```python
from build123d import *

# Parameters (mm, degrees)
F0_W     = 9
F0_H     = 9
F0_H_2   = 432
F1_DEPTH = 18


# Not quite as in the source:
# - a feature names something its author has since deleted; it is built from what else it names


with BuildPart() as f1:
    # F0 (on Front) → F1 (new body)
    with BuildSketch(Plane.XZ):
        with Locations((-1095.5, 71.3756743552)):
            Rectangle(F0_W, F0_H)
        with BuildLine():
            Line((-973.3476458471, -374.1243256448), (-1054.6076226562, -374.1243256448))
            ThreePointArc((-1054.6076226562, -374.1243256448), (-1051.7483407187, -375.721921149), (-1051.265639742, -378.9614896944))
            Line((-1051.265639742, -378.9614896944), (-1098.3606008427, -558.954299013))
            ThreePointArc((-1098.3606008427, -558.954299013), (-1097.4812264988, -563.2754093644), (-1093.523436793, -565.219938755))
            Line((-1093.523436793, -565.219938755), (-1078.8076104242, -565.219938755))
            ThreePointArc((-1078.8076104242, -565.219938755), (-1076.2129629213, -564.4940239596), (-1074.371712623, -562.5270604893))
            Line((-1074.371712623, -562.5270604893), (-977.7835436484, -376.8172039105))
            ThreePointArc((-977.7835436484, -376.8172039105), (-975.94229335, -374.8502404402), (-973.3476458471, -374.1243256448))
        make_face()
        with BuildLine():
            Line((0, -365.1243256448), (-1091, -365.1243256448))
            Line((-1091, -365.1243256448), (-1091, -374.1243256448))
            Line((-1091, -374.1243256448), (-1055, -374.1243256448))
            ThreePointArc((-1055, -374.1243256448), (-1054.8038113281, -374.1191399972), (-1054.6076226562, -374.1243256448))
            Line((-1054.6076226562, -374.1243256448), (-973.3476458471, -374.1243256448))
            Line((-973.3476458471, -374.1243256448), (0, -374.1243256448))
            Line((0, -374.1243256448), (973.3476458471, -374.1243256448))
            Line((973.3476458471, -374.1243256448), (1054.6076226562, -374.1243256448))
            ThreePointArc((1054.6076226562, -374.1243256448), (1054.8038113281, -374.1191399972), (1055, -374.1243256448))
            Line((1055, -374.1243256448), (1100, -374.1243256448))
            Line((1100, -374.1243256448), (1100, 66.8756743552))
            Line((1100, 66.8756743552), (1091, 66.8756743552))
            Line((1091, 66.8756743552), (1091, -365.0378882885))
            Line((1091, -365.0378882885), (1091, -365.1243256448))
            Line((1091, -365.1243256448), (0, -365.1243256448))
        make_face()
        Polygon((0, 75.8756743552), (-1091, 75.8756743552), (-1091, 66.8756743552), (0, 66.8756743552), (1091, 66.8756743552), (1091, 75.8756743552), align=None)
        with Locations((-1095.5, -149.1243256448)):
            Rectangle(F0_W, F0_H_2)
        with Locations((-1095.5, -369.6243256448)):
            Rectangle(F0_W, F0_H)
        with Locations((1095.5, 71.3756743552)):
            Rectangle(F0_W, F0_H)
        with BuildLine():
            ThreePointArc((1051.265639742, -378.9614896944), (1051.7483407187, -375.721921149), (1054.6076226562, -374.1243256448))
            Line((1054.6076226562, -374.1243256448), (973.3476458471, -374.1243256448))
            ThreePointArc((973.3476458471, -374.1243256448), (975.94229335, -374.8502404402), (977.7835436484, -376.8172039105))
            Line((977.7835436484, -376.8172039105), (1074.371712623, -562.5270604893))
            ThreePointArc((1074.371712623, -562.5270604893), (1076.2129629213, -564.4940239596), (1078.8076104242, -565.219938755))
            Line((1078.8076104242, -565.219938755), (1093.523436793, -565.219938755))
            ThreePointArc((1093.523436793, -565.219938755), (1097.4812264988, -563.2754093644), (1098.3606008427, -558.954299013))
            Line((1098.3606008427, -558.954299013), (1051.265639742, -378.9614896944))
        make_face()
        Polygon((0, 66.8756743552), (-1091, 66.8756743552), (-1091, -365.1243256448), (0, -365.1243256448), (1091, -365.1243256448), (1091, -365.0378882885), (1091, 66.8756743552), align=None)
        with BuildLine():
            Line((-1049.9993757457, -21.1739316583), (-1049.9993757457, -21.1230870336))
            Line((-1049.9993757457, -21.1230870336), (-1049.9993757457, -11.824025))
            ThreePointArc((-1049.9993757457, -11.824025), (-1042.6770452754, 5.8536445296), (-1024.9993757457, 13.175975))
            Line((-1024.9993757457, 13.175975), (1024.9993757457, 13.175975))
            ThreePointArc((1024.9993757457, 13.175975), (1042.6770452754, 5.8536445296), (1049.9993757457, -11.824025))
            Line((1049.9993757457, -11.824025), (1049.9993757457, -286.3619962875))
            ThreePointArc((1049.9993757457, -286.3619962875), (1042.6770452754, -304.0396658171), (1024.9993757457, -311.3619962875))
            Line((1024.9993757457, -311.3619962875), (-1024.9993757457, -311.3619962875))
            ThreePointArc((-1024.9993757457, -311.3619962875), (-1042.6770452754, -304.0396658171), (-1049.9993757457, -286.3619962875))
            Line((-1049.9993757457, -286.3619962875), (-1049.9993757457, -21.1739316583))
        make_face(mode=Mode.SUBTRACT)
    extrude(amount=F1_DEPTH)


solid = f1.part
```
Design review of the part built by this model. Coordinates are the model's own, in mm. A direction names the side the tool comes from. Give positions to 0.01 mm unless a question says otherwise; leave off trailing zeros. Order: outer loops, then holes, each group sorted by start corner. A loop starts at its lowest first (then second) coordinate and runs counter-clockwise, first axis right, second up. Notation, with made-up numbers: (-11, -1.5) -> (13, -1.5) arc R19 cw to (13, 30.5) -> close; hole circle Ø6 at (-26.5, -26.75). An arc over 180 degrees is marked (long way). Write item = value, one per line. Start each with the question number.
(1) We need section C-C on y = -11.5. Write out the cut boundary in (x, z).
(2) To check wall thickness, follow line 1 along Z through (x, y) = (-89, -11); line 2 along X through (y, z) = (-1.5, -254.5); line 3 along X through (y, z) = (-16.75, -421.5). State the ranges of each line that lie inside material, in increasing order.
(3) We need section A-A on z = -69. Write out the cut boundary in (x, y), plus the area to 3 significant figures.
(4) Mouldability with a two-part tool opening along X and no side actions: class faces 1 (the face through (-1026.754, -8.874, -470.972)), 2 (the face through (-87, 0, -314)), 3 (the face through (1075.143, -8.874, -470.218)) as +X half, -X half, draft (parallel to the pull), parting line (faces both ways), or undercut.
(5) For pin 1 (3 mm diameter, centred on x = -565, y = -10, fed in from -Z); pin 2 (8 mm diameter, centred on y = -12.5, z = -380, fed in from -X); pin 3 (9 mm diameter, centred on x = 1070, y = -9, fed in from -Z), all flat-tipped, find the tip position at first contact; note any pin that passes through.
(6) We need section B-B on x = 532. Write out the cut boundary in (y, z).
(7) For faces 4 (the face through (1025.4, -8.87, -468.37)), 5 (the face through (-87, -18, -314)), 6 (the face through (-1074.483, -8.874, -467.698)), list the 3-axis set-ups (+Z, -Z, +X, -X, +Y, -Y) from which the entire face can be reached by the end or side of a thin tool; tool diameter is ignored.
Numbers:
q1.outline = (-1100, -374.12) -> (-1055, -374.12) arc R3.71 cw to (-1051.27, -378.96) -> (-1098.36, -558.95) arc R5 ccw to (-1093.52, -565.22) -> (-1078.81, -565.22) arc R5 ccw to (-1074.37, -562.53) -> (-977.78, -376.82) arc R5 cw to (-973.35, -374.12) -> (973.35, -374.12) arc R5 cw to (977.78, -376.82) -> (1074.37, -562.53) arc R5 ccw to (1078.81, -565.22) -> (1093.52, -565.22) arc R5 ccw to (1098.36, -558.95) -> (1051.27, -378.96) arc R3.71 cw to (1055, -374.12) -> (1100, -374.12) -> (1100, 75.88) -> (-1100, 75.88) -> close; hole (-1050, -286.36) arc R25 ccw to (-1025, -311.36) -> (1025, -311.36) arc R25 ccw to (1050, -286.36) -> (1050, -11.82) arc R25 ccw to (1025, 13.18) -> (-1025, 13.18) arc R25 ccw to (-1050, -11.82) -> close
q2.line_1 = -374.12 to -311.36, 13.18 to 75.88
q2.line_2 = -1100 to -1050, 1050 to 1100
q2.line_3 = -1062.4 to -1001.02, 1001.02 to 1062.4
q3.outline = (-1100, -18) -> (-1050, -18) -> (-1050, 0) -> (-1100, 0) -> close; (1050, -18) -> (1100, -18) -> (1100, 0) -> (1050, 0) -> close
q3.area = 1,800 mm^2
q4.face_1 = undercut
q4.face_2 = draft
q4.face_3 = +X half
q5.pin_1 = -374.12
q5.pin_2 = -1052.58
q5.pin_3 = -562.76
q6.outline = (-18, -374.12) -> (0, -374.12) -> (0, -311.36) -> (-18, -311.36) -> close; (-18, 13.18) -> (0, 13.18) -> (0, 75.88) -> (-18, 75.88) -> close
q7.face_4 = -Z, +Y, -Y
q7.face_5 = +Z, -Z, +X, -X, -Y
q7.face_6 = -X, +Y, -Y
